The drawing under review shows one solid part. Ordinate dimensions are in mm from its lowest x, y, z. Coordinates: 2 decimals unless noted, no trailing zeros. Loops run counter-clockwise (first coordinate to the right, second up) from the corner with the lowest first, then second, coordinate; pieces in that order, holes last. Notation, with made-up numbers: M -17.75,30 L 21.25,30 A29 cw 21.25,56 Z; hole C 64,22.5 d10. An arc over 180 degrees is marked long. Put each result on its own line as item: value.
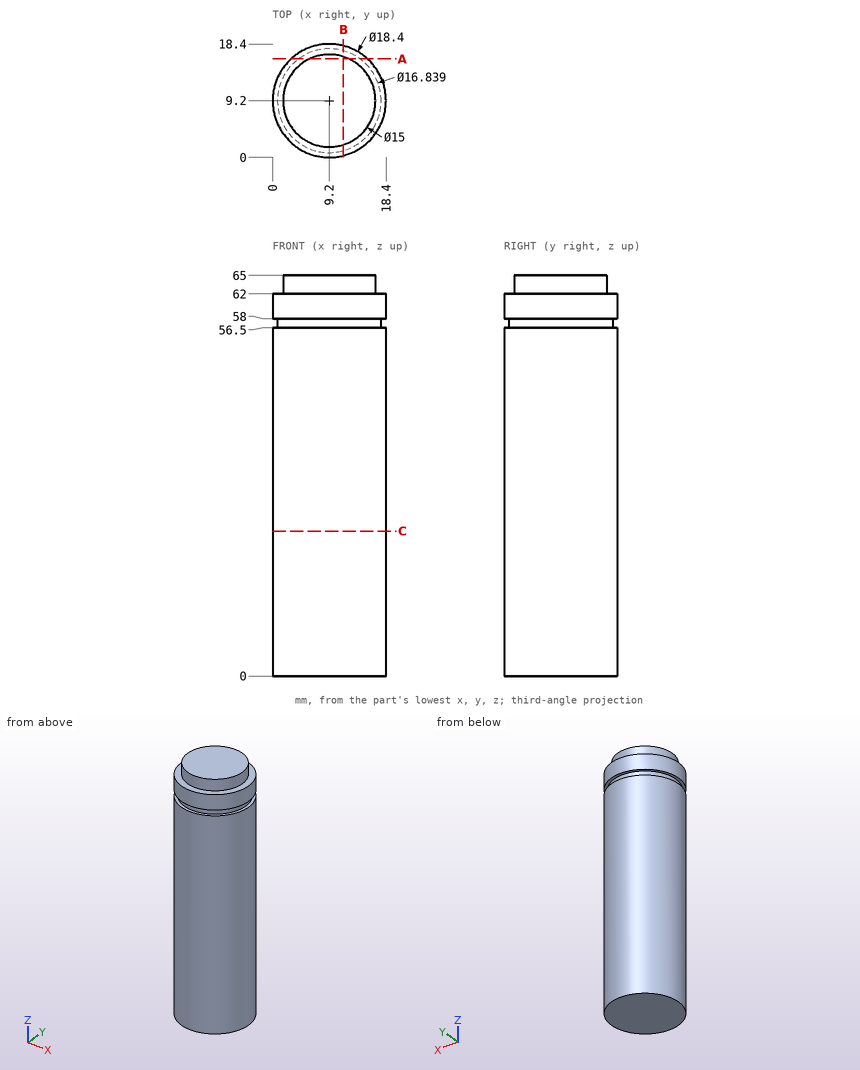
(1) For pin 1 (10 mm diameter, centred on y = 14.5, z = 38.5, fed in from -X) (3 decimals); pin 2 (1.5 mm diameter, centred on x = 14, z = 29.5, fed in from +Y); pin 3 (5 mm diameter, centred on x = 15, z = 54, fed in from -Y), all flat-tipped, find the tip position at first contact; note any pin that passes through.
Determined:
pin 1: stops at x = 0.005
pin 2: stops at y = 17.46
pin 3: stops at y = 0.61
(2) Wall thickness on line 1 along Z through (x, y) = (12.5, 17.75); line 2 along Y through (x, z) = (9.5, 34.5) (3 decimals); line 3 along Y through (x, z) = (12.5, 47): over which ranges is each line inside the solid? List them lowest first. Write a range as [from, to].
Determined:
line 1: z = [0, 56.5], [58, 62]
line 2: y = [0.005, 18.395]
line 3: y = [0.61, 17.79]
(3) Add section A-A (y = 16). Write out the cut boundary in (x, z) (1 decimal), plus the area to 3 significant figures.
Determined:
outline: M 3,0 L 15.4,0 L 15.4,56.5 L 14.2,56.5 L 14.2,58 L 15.4,58 L 15.4,62 L 12.4,62 L 12.4,65 L 6,65 L 6,62 L 3,62 L 3,58 L 4.2,58 L 4.2,56.5 L 3,56.5 Z
area: 784 mm^2
(4) Add section C-C (z = 23.5). Write out the cut boundary in (x, y).
Determined:
outline: C 9.2,9.2 d18.4
(5) Add section B-B (x = 11.5). Write out the cut boundary in (y, z), plus the area to 4 significant figures.
Determined:
outline: M 0.29,0 L 18.11,0 L 18.11,56.5 L 17.3,56.5 L 17.3,58 L 18.11,58 L 18.11,62 L 16.34,62 L 16.34,65 L 2.06,65 L 2.06,62 L 0.29,62 L 0.29,58 L 1.1,58 L 1.1,56.5 L 0.29,56.5 Z
area: 1,145 mm^2
